Read the model definition and answer for the solid it produces. Units are mm, in the model's axes. A direction names the side the tool comes from. Coordinates: 2 decimals unless noted, no trailing zeros. Loops run counter-clockwise (first coordinate to the right, second up) from the corner with the lowest first, then second, coordinate; pieces in that order, holes last. Notation, with made-up numbers: M 39,75.5 L 57,75.5 A19 ccw 57,111.5 Z; hole C 25,-32.5 d10. An arc over 180 degrees is marked long. Put each result on its own line as item: value.
from build123d import *

# Parameters (mm, degrees)
OTHER_10076_5_DEPTH = 0.5
CUT_EXTRUDE1_REACH  = 18.147


# Read off the part's stored shape, not the designer's step: 10076-5
with BuildPart() as part:
    # Other 10076-5 outline → Other 10076-5 (new body)
    with BuildSketch(Plane.XY):
        with BuildLine():
            ThreePointArc((7.573674013, -9.436602245), (7.668819519, -9.359444812), (7.763179028, -9.281328104))
            Line((7.763179028, -9.281328104), (7.919995926, -7.488902759))
            ThreePointArc((7.919995926, -7.488902759), (8.548470738, -6.76266575), (9.110578105, -5.983925684))
            ThreePointArc((9.110578105, -5.983925684), (9.242448569, -5.182849851), (8.736493865, -4.547930843))
            Line((8.736493865, -4.547930843), (8.260223146, -4.3))
            Line((8.260223146, -4.3), (5.774945887, -4.3))
            ThreePointArc((5.774945887, -4.3), (5.659072475, -4.451392897), (5.53923133, -4.5996648))
            Line((5.53923133, -4.5996648), (6.59, -6.419649523))
            ThreePointArc((6.59, -6.419649523), (5.831509763, -7.1157216), (5, -7.722693831))
            Line((5, -7.722693831), (5, -7.841555968))
            ThreePointArc((5, -7.841555968), (0, -9.3), (-5, -7.841555968))
            Line((-5, -7.841555968), (-5, -7.722693831))
            ThreePointArc((-5, -7.722693831), (-5.831509763, -7.1157216), (-6.59, -6.419649523))
            Line((-6.59, -6.419649523), (-5.53923133, -4.5996648))
            ThreePointArc((-5.53923133, -4.5996648), (-5.659072475, -4.451392897), (-5.774945887, -4.3))
            Line((-5.774945887, -4.3), (-8.260223146, -4.3))
            Line((-8.260223146, -4.3), (-10.732831081, -5.58715822))
            ThreePointArc((-10.732831081, -5.58715822), (-10.675718173, -5.6955282), (-10.617511084, -5.803314431))
            Line((-10.617511084, -5.803314431), (-9.055174855, -6.258693914))
            ThreePointArc((-9.055174855, -6.258693914), (-8.704696722, -6.64117368), (-8.882127626, -7.128661083))
            Line((-8.882127626, -7.128661083), (-9.436602245, -7.573674013))
            ThreePointArc((-9.436602245, -7.573674013), (-9.359444812, -7.668819519), (-9.281328104, -7.763179028))
            Line((-9.281328104, -7.763179028), (-7.660171598, -7.905011844))
            ThreePointArc((-7.660171598, -7.905011844), (-7.241809703, -8.211767477), (-7.320727248, -8.724502998))
            Line((-7.320727248, -8.724502998), (-7.777730077, -9.269137762))
            ThreePointArc((-7.777730077, -9.269137762), (-7.683493234, -9.347402405), (-7.588468891, -9.424709008))
            Line((-7.588468891, -9.424709008), (-5.970792243, -9.247544602))
            ThreePointArc((-5.970792243, -9.247544602), (-5.500623999, -9.466787654), (-5.477995427, -9.985067155))
            Line((-5.477995427, -9.985067155), (-5.819964104, -10.608393744))
            ThreePointArc((-5.819964104, -10.608393744), (-5.712269322, -10.666769858), (-5.603989074, -10.724052707))
            Line((-5.603989074, -10.724052707), (-4.05195869, -10.234699407))
            ThreePointArc((-4.05195869, -10.234699407), (-3.548052399, -10.358004491), (-3.424747314, -10.861910782))
            Line((-3.424747314, -10.861910782), (-3.638540174, -11.539975104))
            ThreePointArc((-3.638540174, -11.539975104), (-3.521526102, -11.576219327), (-3.404151099, -11.611277074))
            Line((-3.404151099, -11.611277074), (-1.977410637, -10.828540453))
            ThreePointArc((-1.977410637, -10.828540453), (-1.459131136, -10.851169025), (-1.239888083, -11.321337268))
            Line((-1.239888083, -11.321337268), (-1.317289186, -12.028081692))
            ThreePointArc((-1.317289186, -12.028081692), (-1.195452609, -12.04080118), (-1.073493507, -12.052286575))
            Line((-1.073493507, -12.052286575), (0.173128198, -11.006246762))
            ThreePointArc((0.173128198, -11.006246762), (0.685863719, -10.927329218), (0.992619352, -11.345691113))
            Line((0.992619352, -11.345691113), (1.054584487, -12.053955847))
            ThreePointArc((1.054584487, -12.053955847), (1.176561457, -12.042661796), (1.298417839, -12.030133462))
            Line((1.298417839, -12.030133462), (2.317013814, -10.760989181))
            ThreePointArc((2.317013814, -10.760989181), (2.804501216, -10.583558277), (3.186980982, -10.93403641))
            Line((3.186980982, -10.93403641), (3.38593107, -11.616603238))
            ThreePointArc((3.38593107, -11.616603238), (3.503360927, -11.581729673), (3.620431715, -11.545669067))
            Line((3.620431715, -11.545669067), (4.371857887, -10.10219282))
            ThreePointArc((4.371857887, -10.10219282), (4.815363304, -9.833067127), (5.258868721, -10.10219282))
            Line((5.258868721, -10.10219282), (5.58715822, -10.732831081))
            ThreePointArc((5.58715822, -10.732831081), (5.6955282, -10.675718173), (5.803314431, -10.617511084))
            Line((5.803314431, -10.617511084), (6.258693914, -9.055174855))
            ThreePointArc((6.258693914, -9.055174855), (6.64117368, -8.704696722), (7.128661083, -8.882127626))
            Line((7.128661083, -8.882127626), (7.573674013, -9.436602245))
        make_face()
    extrude(amount=OTHER_10076_5_DEPTH)

    # Sketch1 → Cut-Extrude1 (cut, up to next)
    with BuildSketch(Plane.XY.offset(0.5), mode=Mode.PRIVATE) as cut_extrude1_sk1:
        with BuildLine():
            Line((-9.668418082, -5.033059884), (-10.732831081, -5.58715822))
            ThreePointArc((-10.732831081, -5.58715822), (-10.675718173, -5.6955282), (-10.617511084, -5.803314431))
            Line((-10.617511084, -5.803314431), (-9.055174855, -6.258693914))
            ThreePointArc((-9.055174855, -6.258693914), (-8.908251896, -6.329177308), (-8.791795969, -6.443160998))
            ThreePointArc((-8.791795969, -6.443160998), (-9.25699584, -5.754826497), (-9.668418082, -5.033059884))
        make_face()
    cut_extrude1_tool1 = extrude(cut_extrude1_sk1.sketch, amount=-CUT_EXTRUDE1_REACH, mode=Mode.PRIVATE) & part.part
    add(cut_extrude1_tool1.solids().sort_by_distance((-9.821515, -5.682947, 0.5))[0], mode=Mode.SUBTRACT)


solid = part.part
1) Given pin 1 Ø1 at (x, y) = (3, -7.5) entering from +Z, flat-ended and moving along its own axis, determine where the tip first touches the part or whether it passes through.
Answer list:
pin 1: passes through
2) Which of the six approach directions +Z, -Z, +X, -X, +Y, -Y give full straight-line access (tool end or side, diameter ignored) to faces 1 (the flat face through (-6.07, -5.52, 0.25)), 2 (the cylindrical face through (-9.251, -5.765, 0.254)), 3 (the flat face through (1.801, -11.404, 0.246)), 4 (the flat face through (0, -10, 0.5)), 5 (the cylindrical face through (0.1, -9.3, 0.2))?
Answer list:
face 1: +Z, -Z
face 2: +Z, -Z, -X
face 3: +Z, -Z, -Y
face 4: +Z, +X, -X, +Y, -Y
face 5: +Z, -Z, +Y
3) Straight lines are drawn through the part: line 1 (X direction, y = -11.25, z = 0.1); line 2 (X direction, y = -10, z = 0.2); line 3 (X direction, y = -6, z = 0.35). For each, find the intervals that lie inside material, in ascending order. Write a range as [from, to].
Answer list:
line 1: x = [-3.55, -2.75], [-1.24, -0.12], [0.97, 1.92], [3.28, 3.77]
line 2: x = [-5.49, 4.44], [5.19, 5.98]
line 3: x = [-9.1, -6.35], [6.35, 9.1]
4) Find section A-A, the plane y = -5.5. Write down the section's boundary in (x, z).
Answer list:
outline: M -9.41,0 L -6.06,0 L -6.06,0.5 L -9.41,0.5 Z; M 6.06,0 L 9.27,0 L 9.27,0.5 L 6.06,0.5 Z
5) Determine the mould class of faces 6 (the cylindrical face through (-5.82, -7.125, 0.246)), 7 (the cylindrical face through (8.54, -6.773, 0.246)), 8 (the flat face through (0, -10, 0)), 9 (the cylindrical face through (5.84, -7.11, 0.25)) for opening direction Y: released by +Y, released by -Y, zero draft, split by the parting line, or undercut.
Answer list:
face 6: undercut
face 7: released by -Y
face 8: zero draft
face 9: undercut
6) Find section B-B, the plane x = -0.5. Write down the section's boundary in (y, z).
Answer list:
outline: M -11.57,0 L -9.29,0 L -9.29,0.5 L -11.57,0.5 Z
